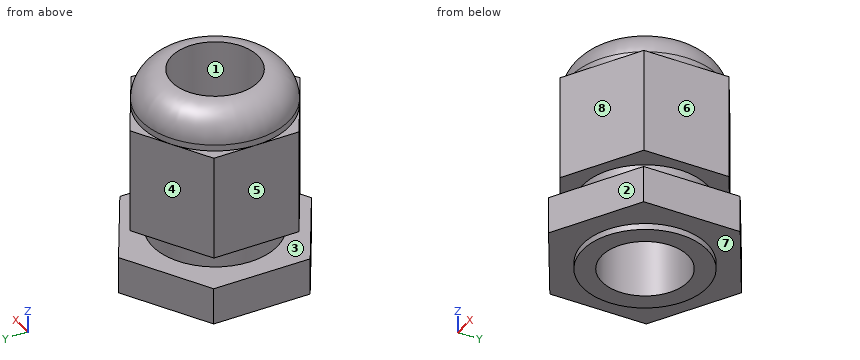
```python
from build123d import *

# Parameters (mm, degrees)
RESSALTO_EXTRUS_O1_DEPTH = 8.5
ESBO_O2_R                = 12
RESSALTO_EXTRUS_O2_DEPTH = 6
FILETE1_R                = 5
ESBO_O3_R                = 10.1
RESSALTO_EXTRUS_O3_DEPTH = 10
RESSALTO_EXTRUS_O4_DEPTH = 6
ESBO_O5_R                = 10.1
RESSALTO_EXTRUS_O5_DEPTH = 1
CORTE_EXTRUS_O1_REACH    = 36
ESBO_O6_R                = 7


with BuildPart() as part:
    # Esboço1 → Ressalto-extrusão1 (new body, symmetric)
    with BuildSketch(Plane.XY):
        Polygon((0, 13.856406461), (-12, 6.92820323), (-12, -6.92820323), (0, -13.856406461), (12, -6.92820323), (12, 6.92820323), align=None)
    extrude(amount=RESSALTO_EXTRUS_O1_DEPTH, both=True)

    # Esboço2 → Ressalto-extrusão2 (add)
    with BuildSketch(Plane.XY.offset(8.5)):
        Circle(ESBO_O2_R)
    extrude(amount=RESSALTO_EXTRUS_O2_DEPTH)

    # Filete1
    filete1_edges = [part.edges().sort_by_distance(p)[0] for p in [
        (-12, 0, 14.5),
    ]]
    fillet(filete1_edges, radius=FILETE1_R)

    # Esboço3 → Ressalto-extrusão3 (add)
    with BuildSketch(Plane(origin=(0, 0, -8.5), x_dir=(-1, 0, 0), z_dir=(0, 0, -1))):
        Circle(ESBO_O3_R)
    extrude(amount=RESSALTO_EXTRUS_O3_DEPTH)

    # Esboço4 → Ressalto-extrusão4 (add)
    with BuildSketch(Plane(origin=(0, 0, -18.5), x_dir=(-1, 0, 0), z_dir=(0, 0, -1))):
        Polygon((0, 15.703927322), (-13.6, 7.851963661), (-13.6, -7.851963661), (0, -15.703927322), (13.6, -7.851963661), (13.6, 7.851963661), align=None)
    extrude(amount=-RESSALTO_EXTRUS_O4_DEPTH)

    # Esboço5 → Ressalto-extrusão5 (add)
    with BuildSketch(Plane(origin=(0, 0, -18.5), x_dir=(-1, 0, 0), z_dir=(0, 0, -1))):
        Circle(ESBO_O5_R)
    extrude(amount=RESSALTO_EXTRUS_O5_DEPTH)

    # Esboço6 → Corte-extrusão1 (cut, up to next)
    with BuildSketch(Plane.XY.offset(14.5), mode=Mode.PRIVATE) as corte_extrus_o1_sk1:
        Circle(ESBO_O6_R)
    corte_extrus_o1_tool1 = extrude(corte_extrus_o1_sk1.sketch, amount=-CORTE_EXTRUS_O1_REACH, mode=Mode.PRIVATE) & part.part
    add(corte_extrus_o1_tool1.solids().sort_by_distance((0, 0, 14.5))[0], mode=Mode.SUBTRACT)


solid = part.part
```
Could you check a few things on this model? Use its own coordinates, in mm. Face numbers are marked on the shaded views. A direction names the side the tool comes from. Coordinates: 2 decimals unless noted, no trailing zeros. Write each loop counter-clockwise with the first axis right and the second up, starting at its lowest first coordinate (ties: lowest second). Pieces come first, ordered by that corner, then holes. Notation, with made-up numbers: (15, -38) -> (50, -38) arc R26 ccw to (50, 1) -> close; hole circle Ø9 at (14.5, -26.5). An arc over 180 degrees is marked (long way). One line per question, with ' | ' between items. Start each with the question number.
1. If we section it at B-B (z = -16): Please give me the cut outline in (x, y).
2. Please list where these lines run through material, in increasing order: line 1 along Y through (x, z) = (0, 7.5); line 2 along Y through (x, z) = (0, -10); line 3 along X through (y, z) = (-6, 7).
3. Thinking about a two-plate mould opening in X: for the marked faces 1, 2 and 3, which applies, pulls with the +X half, pulls with the -X half, needs draft (parallel to the pull), parting line crosses it, or undercut?
4. If we section it at D-D (z = -12): Please give me the cut outline in (x, y).
5. Will these pins go through, and if not, where does the flat tip stop? P1, Ø10, axis at x = -6.5, z = -14.5, coming from the -Y side; P2, Ø5, axis at x = 10, z = 6.5, coming from the -Y side; P3, Ø3, axis at x = 5.5, y = 6, coming from the +Z side; P4, Ø1.8, axis at x = 8.5, y = -8, coming from the +Z side.
6. If we section it at A-A (z = 5.5): Please give me the cut outline in (x, y), and give its area (3 significant figures).
7. If we section it at C-C (z = 9): Please give me the cut outline in (x, y), and give its area (3 significant figures).
8. For the marked faces 4, 5, 6, 7 and 8, which set-ups out of +Z, -Z, +X, -X, +Y, -Y let a thin tool reach every point of the face, with its end or its side?
Return value:
1) outline: (-13.6, -7.85) -> (0, -15.7) -> (13.6, -7.85) -> (13.6, 7.85) -> (0, 15.7) -> (-13.6, 7.85) -> close; hole circle Ø14 at (0, 0)
2) line 1: y = -13.86 to -7, 7 to 13.86 | line 2: y = -10.1 to -7, 7 to 10.1 | line 3: x = -12 to -3.61, 3.61 to 12
3) face 1: undercut | face 2: pulls with the +X half | face 3: needs draft
4) outline: circle Ø20.2 at (0, 0); hole circle Ø14 at (0, 0)
5) P1: stops at y = -14.84 | P2: stops at y = -9.53 | P3: stops at z = 14.5 | P4: stops at z = 12.78
6) outline: (-12, -6.93) -> (0, -13.86) -> (12, -6.93) -> (12, 6.93) -> (0, 13.86) -> (-12, 6.93) -> close; hole circle Ø14 at (0, 0) | area: 345 mm²
7) outline: circle Ø24 at (0, 0); hole circle Ø14 at (0, 0) | area: 298 mm²
8) face 4: +Z, -X, +Y | face 5: +Z, -X, +Y, -Y | face 6: +Z, +X, +Y, -Y | face 7: -Z | face 8: +Z, +X, -Y
